Verification items for the finished model (mm, model axes). Give positions to 0.01 mm unless a question says otherwise; leave off trailing zeros. One line per item, written item: value. Start each with the question number.
1. Gauge pin test, flat ends, axial feed: pin 1 (1.5 mm diameter, centred on y = 106, z = 9, fed in from -X); pin 2 (20.5 mm diameter, centred on x = 127, y = 76.2, fed in from -Z); pin 3 (6 mm diameter, centred on y = -198, z = 10.5, fed in from +X). Record the tip position at first contact, or that the pin passes through.
2. Scan lines: L1, parallel to Y at x = 0, z = 5.5; L2, parallel to X at y = -77, z = 5.5; L3, parallel to X at y = 207, z = 5.5. Record each from-to range of solid material in increasing order. Write a range as [from, to].
3. Mould release check, pull along Y, two halves, no side actions. Record for faces 1 (the cylindrical face through (49.147, -190.608, 6.439)), 2 (the flat face through (-2, 53, 12.7)): pulls with the +Y half, pulls with the -Y half, needs draft (parallel to the pull), parting line crosses it, or undercut.
4. Sectioned sample at A-A (z = 6.75). Count the separate pieces of the cut face and the enclosed holes in it, plus the area to 3 significant figures.
from build123d import *

# Parameters (mm, degrees)
SKETCH2_RX          = 254
SKETCH2_RY          = 152.143434343
BOSS_EXTRUDE2_DEPTH = 12.7
SKETCH3_R           = 50.8
SKETCH3_R_2         = 12.7
SKETCH3_R_3         = 6.35
CUT_EXTRUDE1_DEPTH  = 12.7


with BuildPart() as part:
    # Sketch2 → Boss-Extrude2 (new body)
    with BuildSketch(Plane(origin=(0, 0, 0), x_dir=(0, 1, 0), z_dir=(0, 0, 1))):
        with Locations((0, 0)):
            Ellipse(SKETCH2_RX, SKETCH2_RY)
    extrude(amount=BOSS_EXTRUDE2_DEPTH)

    # Sketch3 → Cut-Extrude1 (cut)
    with BuildSketch(Plane.XY.offset(12.7)):
        Circle(SKETCH3_R)
        with Locations((-50.8, 203.2)):
            Circle(SKETCH3_R_2)
        with Locations((50.8, 203.2)):
            Circle(SKETCH3_R_2)
        with Locations((127, 76.2)):
            Circle(SKETCH3_R_2)
        with Locations((127, -76.2)):
            Circle(SKETCH3_R_2)
        with Locations((-50.8, -203.2)):
            Circle(SKETCH3_R_2)
        with Locations((50.8, -203.2)):
            Circle(SKETCH3_R_2)
        with Locations((-127, 76.2)):
            Circle(SKETCH3_R_2)
        with Locations((-127, -76.2)):
            Circle(SKETCH3_R_2)
        with Locations((0, 76.2)):
            Circle(SKETCH3_R_3)
        with Locations((0, -76.2)):
            Circle(SKETCH3_R_3)
        with Locations((0, 152.4)):
            Circle(SKETCH3_R_3)
        with Locations((0, -152.4)):
            Circle(SKETCH3_R_3)
    extrude(amount=-CUT_EXTRUDE1_DEPTH, mode=Mode.SUBTRACT)


solid = part.part
Results are:
1. pin 1: stops at x = -138.47
1. pin 2: passes through
1. pin 3: stops at x = 97.49
2. L1: y = [-254, -158.75], [-146.05, -82.55], [-69.85, -50.8], [50.8, 69.85], [82.55, 146.05], [158.75, 254]
2. L2: x = [-144.98, -139.67], [-114.33, -6.3], [6.3, 114.33], [139.67, 144.98]
2. L3: x = [-88.17, -62.92], [-38.68, 38.68], [62.92, 88.17]
3. face 1: undercut
3. face 2: needs draft
4. separate pieces: 1
4. enclosed holes: 13
4. area: 109,000 mm^2
